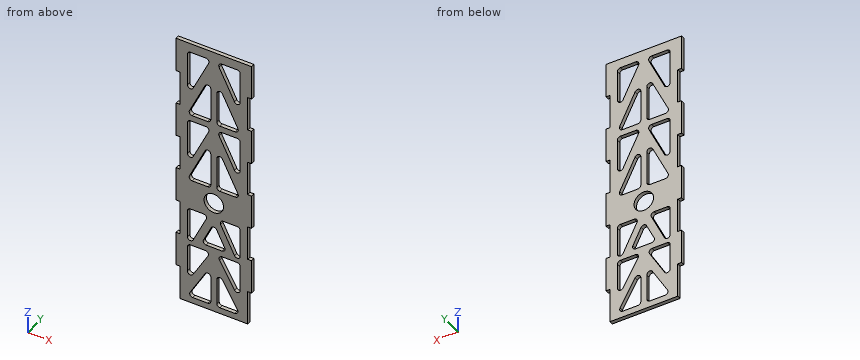
from build123d import *

# Parameters (mm, degrees)
SKETCH1_R           = 8.1915
BOSS_EXTRUDE1_DEPTH = 3.175


with BuildPart() as part:
    # Sketch1 → Boss-Extrude1 (new body)
    with BuildSketch(Plane(origin=(0, -9.743731804, 0), x_dir=(1, 0, 0), z_dir=(0, 1, 0))):
        Polygon((-31.75, 143.175862399), (-28.575, 143.175862399), (-28.575, 171.750862399), (28.575, 171.750862399), (28.575, 143.175862399), (31.75, 143.175862399), (31.75, 114.600862399), (28.575, 114.600862399), (28.575, 86.025862399), (31.75, 86.025862399), (31.75, 57.450862399), (28.575, 57.450862399), (28.575, 28.875862399), (31.75, 28.875862399), (31.75, 0.300862399), (28.575, 0.300862399), (28.575, -28.274137601), (31.75, -28.274137601), (31.75, -56.849137601), (-31.75, -56.849137601), (-31.75, -28.274137601), (-28.575, -28.274137601), (-28.575, 0.300862399), (-31.75, 0.300862399), (-31.75, 28.875862399), (-28.575, 28.875862399), (-28.575, 57.450862399), (-31.75, 57.450862399), (-31.75, 86.025862399), (-28.575, 86.025862399), (-28.575, 114.600862399), (-31.75, 114.600862399), align=None)
        with Locations((0, 76.500862399)):
            Circle(SKETCH1_R, mode=Mode.SUBTRACT)
        with BuildLine():
            Line((-17.769774531, 166.670862399), (-5.08, 166.670862399))
            ThreePointArc((-5.08, 166.670862399), (-3.283948776, 165.926913623), (-2.54, 164.130862399))
            Line((-2.54, 164.130862399), (-2.54, 142.693779868))
            ThreePointArc((-2.54, 142.693779868), (-4.409257974, 140.243942091), (-7.265752074, 141.399914392))
            Line((-7.265752074, 141.399914392), (-19.955526605, 162.836996923))
            ThreePointArc((-19.955526605, 162.836996923), (-19.976357671, 165.388873069), (-17.769774531, 166.670862399))
        make_face(mode=Mode.SUBTRACT)
        with BuildLine():
            Line((2.54, 164.130862399), (2.54, 142.693779868))
            ThreePointArc((2.54, 142.693779868), (4.409257974, 140.243942091), (7.265752074, 141.399914392))
            Line((7.265752074, 141.399914392), (19.955526605, 162.836996923))
            ThreePointArc((19.955526605, 162.836996923), (19.976357671, 165.388873069), (17.769774531, 166.670862399))
            Line((17.769774531, 166.670862399), (5.08, 166.670862399))
            ThreePointArc((5.08, 166.670862399), (3.283948776, 165.926913623), (2.54, 164.130862399))
        make_face(mode=Mode.SUBTRACT)
        with BuildLine():
            Line((-22.225, 144.92794493), (-22.225, 123.490862399))
            ThreePointArc((-22.225, 123.490862399), (-21.481051224, 121.694811175), (-19.685, 120.950862399))
            Line((-19.685, 120.950862399), (-6.995225469, 120.950862399))
            ThreePointArc((-6.995225469, 120.950862399), (-4.788642329, 122.232851729), (-4.809473395, 124.784727875))
            Line((-4.809473395, 124.784727875), (-17.499247926, 146.221810406))
            ThreePointArc((-17.499247926, 146.221810406), (-20.355742026, 147.377782707), (-22.225, 144.92794493))
        make_face(mode=Mode.SUBTRACT)
        with BuildLine():
            Line((4.809473395, 124.784727875), (17.499247926, 146.221810406))
            ThreePointArc((17.499247926, 146.221810406), (20.355742026, 147.377782707), (22.225, 144.92794493))
            Line((22.225, 144.92794493), (22.225, 123.490862399))
            ThreePointArc((22.225, 123.490862399), (21.481051224, 121.694811175), (19.685, 120.950862399))
            Line((19.685, 120.950862399), (6.995225469, 120.950862399))
            ThreePointArc((6.995225469, 120.950862399), (4.788642329, 122.232851729), (4.809473395, 124.784727875))
        make_face(mode=Mode.SUBTRACT)
        with BuildLine():
            Line((5.749780192, 92.89598746), (17.422858074, 115.75598746))
            ThreePointArc((17.422858074, 115.75598746), (20.279036829, 117.070421114), (22.225, 114.600862399))
            Line((22.225, 114.600862399), (22.225, 91.740862399))
            ThreePointArc((22.225, 91.740862399), (21.481051224, 89.944811175), (19.685, 89.200862399))
            Line((19.685, 89.200862399), (8.011922118, 89.200862399))
            ThreePointArc((8.011922118, 89.200862399), (5.845632934, 90.414668155), (5.749780192, 92.89598746))
        make_face(mode=Mode.SUBTRACT)
        with BuildLine():
            Line((-6.372736394, 92.844195759), (-17.397150465, 115.704195759))
            ThreePointArc((-17.397150465, 115.704195759), (-20.250889645, 117.077022513), (-22.225, 114.600862399))
            Line((-22.225, 114.600862399), (-22.225, 91.740862399))
            ThreePointArc((-22.225, 91.740862399), (-21.481051224, 89.944811175), (-19.685, 89.200862399))
            Line((-19.685, 89.200862399), (-8.66058593, 89.200862399))
            ThreePointArc((-8.66058593, 89.200862399), (-6.509531917, 90.390097196), (-6.372736394, 92.844195759))
        make_face(mode=Mode.SUBTRACT)
        with BuildLine():
            Line((5.08, 63.800862399), (18.076004066, 63.800862399))
            ThreePointArc((18.076004066, 63.800862399), (20.24229325, 62.587056643), (20.338145992, 60.105737338))
            Line((20.338145992, 60.105737338), (7.342141926, 34.654981681))
            ThreePointArc((7.342141926, 34.654981681), (4.485963171, 33.340548027), (2.54, 35.810106741))
            Line((2.54, 35.810106741), (2.54, 61.260862399))
            ThreePointArc((2.54, 61.260862399), (3.283948776, 63.056913623), (5.08, 63.800862399))
        make_face(mode=Mode.SUBTRACT)
        with BuildLine():
            Line((-5.08, 63.800862399), (-18.180124412, 63.800862399))
            ThreePointArc((-18.180124412, 63.800862399), (-20.331178425, 62.611627602), (-20.467973948, 60.157529039))
            Line((-20.467973948, 60.157529039), (-7.367849535, 32.993378441))
            ThreePointArc((-7.367849535, 32.993378441), (-4.514110355, 31.620551687), (-2.54, 34.096711801))
            Line((-2.54, 34.096711801), (-2.54, 61.260862399))
            ThreePointArc((-2.54, 61.260862399), (-3.283948776, 63.056913623), (-5.08, 63.800862399))
        make_face(mode=Mode.SUBTRACT)
        with BuildLine():
            Line((17.422858074, 40.433585982), (4.426854008, 14.982830325))
            ThreePointArc((4.426854008, 14.982830325), (4.52270675, 12.50151102), (6.688995934, 11.287705264))
            Line((6.688995934, 11.287705264), (19.685, 11.287705264))
            ThreePointArc((19.685, 11.287705264), (21.481051224, 12.03165404), (22.225, 13.827705264))
            Line((22.225, 13.827705264), (22.225, 39.278460922))
            ThreePointArc((22.225, 39.278460922), (20.279036829, 41.748019636), (17.422858074, 40.433585982))
        make_face(mode=Mode.SUBTRACT)
        with BuildLine():
            Line((-22.225, 40.991855862), (-22.225, 13.827705264))
            ThreePointArc((-22.225, 13.827705264), (-21.481051224, 12.03165404), (-19.685, 11.287705264))
            Line((-19.685, 11.287705264), (-6.584875588, 11.287705264))
            ThreePointArc((-6.584875588, 11.287705264), (-4.433821575, 12.476940061), (-4.297026052, 14.931038624))
            Line((-4.297026052, 14.931038624), (-17.397150465, 42.095189222))
            ThreePointArc((-17.397150465, 42.095189222), (-20.250889645, 43.468015976), (-22.225, 40.991855862))
        make_face(mode=Mode.SUBTRACT)
        with BuildLine():
            Line((-18.180124412, 6.207705264), (-5.08, 6.207705264))
            ThreePointArc((-5.08, 6.207705264), (-3.283948776, 5.463756488), (-2.54, 3.667705264))
            Line((-2.54, 3.667705264), (-2.54, -23.496445334))
            ThreePointArc((-2.54, -23.496445334), (-4.514110355, -25.972605448), (-7.367849535, -24.599778694))
            Line((-7.367849535, -24.599778694), (-20.467973948, 2.564371904))
            ThreePointArc((-20.467973948, 2.564371904), (-20.331178425, 5.018470467), (-18.180124412, 6.207705264))
        make_face(mode=Mode.SUBTRACT)
        with BuildLine():
            Line((2.54, 3.667705264), (2.54, -21.783050394))
            ThreePointArc((2.54, -21.783050394), (4.485963171, -24.252609108), (7.342141926, -22.938175454))
            Line((7.342141926, -22.938175454), (20.338145992, 2.512580203))
            ThreePointArc((20.338145992, 2.512580203), (20.24229325, 4.993899508), (18.076004066, 6.207705264))
            Line((18.076004066, 6.207705264), (5.08, 6.207705264))
            ThreePointArc((5.08, 6.207705264), (3.283948776, 5.463756488), (2.54, 3.667705264))
        make_face(mode=Mode.SUBTRACT)
        with BuildLine():
            Line((4.426854008, -45.53401254), (17.422858074, -20.083256883))
            ThreePointArc((17.422858074, -20.083256883), (20.279036829, -18.768823229), (22.225, -21.238381943))
            Line((22.225, -21.238381943), (22.225, -46.689137601))
            ThreePointArc((22.225, -46.689137601), (21.481051224, -48.485188825), (19.685, -49.229137601))
            Line((19.685, -49.229137601), (6.688995934, -49.229137601))
            ThreePointArc((6.688995934, -49.229137601), (4.52270675, -48.015331845), (4.426854008, -45.53401254))
        make_face(mode=Mode.SUBTRACT)
        with BuildLine():
            Line((-17.397150465, -18.421653643), (-4.297026052, -45.585804241))
            ThreePointArc((-4.297026052, -45.585804241), (-4.433821575, -48.039902804), (-6.584875588, -49.229137601))
            Line((-6.584875588, -49.229137601), (-19.685, -49.229137601))
            ThreePointArc((-19.685, -49.229137601), (-21.481051224, -48.485188825), (-22.225, -46.689137601))
            Line((-22.225, -46.689137601), (-22.225, -19.524987003))
            ThreePointArc((-22.225, -19.524987003), (-20.250889645, -17.048826889), (-17.397150465, -18.421653643))
        make_face(mode=Mode.SUBTRACT)
        with BuildLine():
            Line((6.89223147, 115.870862399), (-6.382799442, 115.870862399))
            ThreePointArc((-6.382799442, 115.870862399), (-8.533853455, 114.681627602), (-8.670648977, 112.227529039))
            Line((-8.670648977, 112.227529039), (-2.222824791, 98.857452412))
            ThreePointArc((-2.222824791, 98.857452412), (0.036114273, 97.420950308), (2.32716667, 98.805660711))
            Line((2.32716667, 98.805660711), (9.154373397, 112.175737338))
            ThreePointArc((9.154373397, 112.175737338), (9.058520654, 114.657056643), (6.89223147, 115.870862399))
        make_face(mode=Mode.SUBTRACT)
    extrude(amount=BOSS_EXTRUDE1_DEPTH)


solid = part.part
The listing builds one solid part. Answer for the finished solid, in the listing's coordinates (mm). Give positions to 0.01 mm unless a question says otherwise; leave off trailing zeros. Write each loop counter-clockwise with the first axis right and the second up, starting at its lowest first coordinate (ties: lowest second). Pieces come first, ordered by that corner, then holes.
1) Section A-A (z = -101.5) is taken. Write down the section's boundary in (x, y) (3 decimals).
2) Section B-B (x = 0) is taken. Write down the section's boundary in (y, z), and give its area (3 significant figures).
3) Section C-C (z = 34) is taken. Count the separate pieces of the cut face and the enclosed holes in it, and give its area (3 significant figures).
4) Given P1, Ø1, axis at y = -8.5, z = -98, coming from the -X side (3 decimals); P2, Ø1.6, axis at y = -8.5, z = -156.5, coming from the +X side (3 decimals); P3, Ø1.6, axis at x = -30, y = -8.5, coming from the -Z side, each flat-ended and moving along its own axis, determine where each tip first touches the part or whether it passes through.
5) Find the intervals of material crossed by L1, parallel to Z at x = 0, y = -8.25; L2, parallel to X at y = -7.6, z = -123; L3, parallel to X at y = -7.3, z = -43 (3 decimals), in increasing order.
Response:
1. outline: (-28.575, -9.744) - (-22.225, -9.744) - (-22.225, -6.569) - (-28.575, -6.569) - close; (-10.547, -9.744) - (-3.497, -9.744) - (-3.497, -6.569) - (-10.547, -6.569) - close; (3.703, -9.744) - (10.143, -9.744) - (10.143, -6.569) - (3.703, -6.569) - close; (22.225, -9.744) - (28.575, -9.744) - (28.575, -6.569) - (22.225, -6.569) - close
2. outline: (-9.74, -171.75) - (-6.57, -171.75) - (-6.57, -115.87) - (-9.74, -115.87) - close; (-9.74, -97.42) - (-6.57, -97.42) - (-6.57, -84.69) - (-9.74, -84.69) - close; (-9.74, -68.31) - (-6.57, -68.31) - (-6.57, 56.85) - (-9.74, 56.85) - close
2. area: 615 mm2
3. separate pieces: 3
3. enclosed holes: 0
3. area: 125 mm2
4. P1: stops at x = -28.575
4. P2: stops at x = 28.575
4. P3: stops at z = -143.18
5. L1: z = -171.75 to -115.87, -97.42 to -84.69, -68.31 to 56.85
5. L2: x = -31.75 to -22.18, -4.5 to 4.5, 22.18 to 31.75
5. L3: x = -28.575 to -21.24, -18.13 to -12.194, -2.54 to 2.54, 11.603 to 28.575
